from build123d import *

# Parameters (mm, degrees)
F1_DEPTH = 2
F3_DEPTH = 8
F4_R     = 1.5
F5_DEPTH = 8
F6_SIZE  = 1


with BuildPart() as f1:
    # F0 (on Top) → F1 (new body)
    with BuildSketch(Plane.XY):
        with BuildLine():
            Line((-10.922433, 40.600829), (-37.822433, 23.600829))
            Line((-37.822433, 23.600829), (-37.822433, -26.399171))
            Line((-37.822433, -26.399171), (-10.922433, -43.399171))
            ThreePointArc((-10.922433, -43.399171), (-0.822433, -39.026117), (9.277567, -43.399171))
            Line((9.277567, -43.399171), (36.177567, -26.399171))
            Line((36.177567, -26.399171), (36.177567, 23.600829))
            Line((36.177567, 23.600829), (9.277567, 40.600829))
            ThreePointArc((9.277567, 40.600829), (-0.822433, 36.227775), (-10.922433, 40.600829))
        make_face()
    extrude(amount=-F1_DEPTH)

    # F2 (on Top) → F3 (join)
    with BuildSketch(Plane.XY):
        Polygon((36.177567, -15.736748), (36.177567, 23.600829), (9.277567, 40.600829), (9.277567, 38.826394), (34.677567, 22.774349), (34.677567, -18.295043), (34.677567, -25.572692), (9.277567, -41.624736), (9.277567, -43.399171), (36.177567, -26.399171), align=None)
        Polygon((-10.922433, 38.826394), (-10.922433, 40.600829), (-37.822433, 23.600829), (-37.822433, -26.399171), (-10.922433, -43.399171), (-10.922433, -41.624736), (-31.431845, -28.663398), (-36.322433, -25.572692), (-36.322433, 22.774349), align=None)
    extrude(amount=F3_DEPTH)

    # F4 (on face) → F5 (join)
    with BuildSketch(Plane.XY):
        with Locations((-0.822433, -25.572692)):
            Circle(F4_R)
        with Locations((-0.822433, -1.399171)):
            Circle(F4_R)
        with Locations((16.677567, -10.911981)):
            Circle(F4_R)
        with Locations((16.677567, 11.862593)):
            Circle(F4_R)
        with Locations((-18.322433, 11.862593)):
            Circle(F4_R)
        with Locations((-18.322433, -10.911981)):
            Circle(F4_R)
        Polygon((-3.420509, 21.274349), (1.775643, 21.274349), (-0.822433, 25.774349), align=None)
    extrude(amount=F5_DEPTH)

    # F6
    f6_edges = [f1.edges().sort_by_distance(p)[0] for p in [
        (-10.922433, 38.826394, 4),
        (9.277567, 38.826394, 4),
        (-10.922433, -41.624736, 4),
        (9.277567, -41.624736, 4),
    ]]
    chamfer(f6_edges, length=F6_SIZE)


solid = f1.part
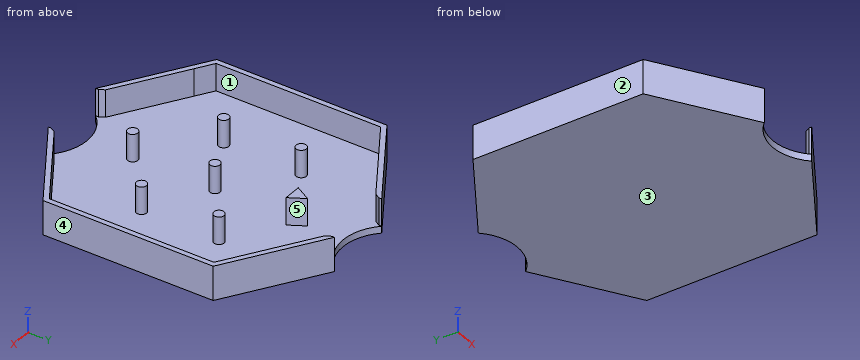
Part model, mm, in its own coordinate system. Face numbers are marked on the shaded views. A direction names the side the tool comes from. Round coordinates to 2 decimals unless told otherwise and drop trailing zeros. Loops run counter-clockwise (first coordinate to the right, second up) from the corner with the lowest first, then second, coordinate; pieces in that order, holes last. Notation, with made-up numbers: (40, 3) - (52, 3) arc R27 ccw to (52, 32) - close; hole circle Ø7 at (76.5, -6.5). An arc over 180 degrees is marked (long way). Answer as a JSON object with one key per item and string values.
Item 1: Pin check, flat tips, straight feed: pin 1 (2.5 mm diameter, centred on x = -0.5, z = 4, fed in from -Y); pin 2 (1 mm diameter, centred on y = -29.5, z = -0.5, fed in from -X); pin 3 (1.5 mm diameter, centred on x = -26.5, y = -15.5, fed in from +Z). Stop position of each tip, or through.
Output:
{"pin 1": "y = -27.07", "pin 2": "x = -33.71", "pin 3": "z = 0"}
Item 2: Band-saw the part on C-C on x = -27. List the corners of the cut face in (y, z), plus the area to 3 significant figures.
Output:
{"outline": "(-33.24, -2) - (30.44, -2) - (30.44, 8) - (28.67, 8) - (28.67, 0) - (-31.46, 0) - (-31.46, 8) - (-33.24, 8) - close", "area": "156 mm2"}
Item 3: Tool access for the marked faces 1 and 2: list every direction of +Z, -Z, +X, -X, +Y, -Y with a clear straight run to the whole face (end or side of a thin tool).
Output:
{"face 1": "+Z", "face 2": "+Z, -Z, -X, +Y, -Y"}
Item 4: Wall check: L1, parallel to X at y = 19, z = 2.5; L2, parallel to Y at x = -19.5, z = 5.25; L3, parallel to X at y = 25.5, z = 3.25. Give the ranges that are in metal, low to high.
Output:
{"L1": "-37.82 to -36.32, 34.68 to 36.18", "L2": "-37.98 to -36.2, -11.84 to -9.98, 10.93 to 12.79, 33.41 to 35.18", "L3": "-34.82 to -32.01, -0.98 to -0.66, 30.36 to 33.17"}
Item 5: Band-saw the part on A-A on y = -5. List the corners of the cut face in (x, z), plus the area to 3 significant figures.
Output:
{"outline": "(-37.82, -2) - (36.18, -2) - (36.18, 8) - (34.68, 8) - (34.68, 0) - (-36.32, 0) - (-36.32, 8) - (-37.82, 8) - close", "area": "172 mm2"}
Item 6: Pull direction X, two halves, no side cores. Call the marked faces 3, 4 and 5: pulls with the +X half, pulls with the -X half, needs draft (parallel to the pull), parting line crosses it, or undercut.
Output:
{"face 3": "needs draft", "face 4": "pulls with the +X half", "face 5": "undercut"}
Item 7: Band-saw the part on B-B on z = 2. State how many separate pieces and enclosed holes the cut face has, plus the area to 3 significant figures.
Output:
{"separate pieces": "9", "enclosed holes": "0", "area": "386 mm2"}
